from build123d import *

# Parameters (mm, degrees)
F0_W     = 100
F0_H     = 40
F1_DEPTH = 10
F2_R     = 5
F3_DEPTH = 10
F4_W     = 30
F4_H     = 40
F5_DEPTH = 10
F6_W     = 30
F6_H     = 20
F7_DEPTH = 10


with BuildPart() as f1:
    # F0 (on Top) → F1 (new body)
    with BuildSketch(Plane.XY):
        with Locations((40, 0)):
            Rectangle(F0_W, F0_H)
    extrude(amount=F1_DEPTH)

    # F2 (on face) → F3 (cut, through all)
    with BuildSketch(Plane.XY.offset(10)):
        Circle(F2_R)
    extrude(amount=-F3_DEPTH, mode=Mode.SUBTRACT)

    # F4 (on face) → F5 (join)
    with BuildSketch(Plane.XY.offset(10)):
        with Locations((75, 0)):
            Rectangle(F4_W, F4_H)
    extrude(amount=F5_DEPTH)

    # F6 (on face) → F7 (cut)
    with BuildSketch(Plane.XY.offset(20)):
        with Locations((75, 0)):
            Rectangle(F6_W, F6_H)
    extrude(amount=-F7_DEPTH, mode=Mode.SUBTRACT)


solid = f1.part
Can you work these out from the model? Positions are in its coordinate system, mm. A direction names the side the tool comes from. Give positions to 0.01 mm unless a question says otherwise; leave off trailing zeros. Loops run counter-clockwise (first coordinate to the right, second up) from the corner with the lowest first, then second, coordinate; pieces in that order, holes last. Notation, with made-up numbers: (6.25, 46) - (14.25, 46) arc R20 ccw to (14.25, 75) - close; hole circle Ø3 at (79, 20.5). An arc over 180 degrees is marked (long way). Return JSON: item names as keys, results as strings.
1. For faces 1 (the face through (-10, 0, 5)), 2 (the face through (75, -10, 15)), 3 (the face through (60, -15, 15)), which set-ups out of +Z, -Z, +X, -X, +Y, -Y let a thin tool reach every point of the face, with its end or its side?
Output values:
{"face 1": "+Z, -Z, -X, +Y, -Y", "face 2": "+Z, +X, -X", "face 3": "+Z, -X, +Y, -Y"}
2. I want a section at A-A on x = 4. Please give me the cut outline in (y, z), and give its area (3 significant figures).
Output values:
{"outline": "(-20, 0) - (-3, 0) - (-3, 10) - (-20, 10) - close; (3, 0) - (20, 0) - (20, 10) - (3, 10) - close", "area": "340 mm²"}
3. I want a section at B-B on y = 0. Please give me the cut outline in (x, z), and give its area (3 significant figures).
Output values:
{"outline": "(-10, 0) - (-5, 0) - (-5, 10) - (-10, 10) - close; (5, 0) - (90, 0) - (90, 10) - (5, 10) - close", "area": "900 mm²"}
4. I'm going to push flat-ended pins straight in: pin 1 Ø11.5 at (x, y) = (0, 0) entering from +Z; pin 2 Ø8 at (y, z) = (7.5, 14.5) entering from -X. Where does each tip first touch, or does it pass through?
Output values:
{"pin 1": "stops at z = 10", "pin 2": "stops at x = 60"}
5. If I drill on line 1 (Y direction, x = 0, z = 7.75); line 2 (Y direction, x = 63.5, z = 12.25); line 3 (Z direction, x = 76, y = -7.5), over which ranges is the centre line in solid material (lowest first)?
Output values:
{"line 1": "y = -20 to -5, 5 to 20", "line 2": "y = -20 to -10, 10 to 20", "line 3": "z = 0 to 10"}
6. We'd pull the mould along Y, two halves only. Please class faces 4 (the face through (-1.08, -4.88, 5.07)), 5 (the face through (75, -15, 20)), 6 (the face through (50, 20, 8)): +Y half, -Y half, draft (parallel to the pull), parting line (faces both ways), or undercut.
Output values:
{"face 4": "undercut", "face 5": "draft", "face 6": "+Y half"}
7. I want a section at D-D on x = 83. Please give me the cut outline in (y, z), and give its area (3 significant figures).
Output values:
{"outline": "(-20, 0) - (20, 0) - (20, 20) - (10, 20) - (10, 10) - (-10, 10) - (-10, 20) - (-20, 20) - close", "area": "600 mm²"}
8. I want a section at C-C on z = 4. Please give me the cut outline in (x, y), and give its area (3 significant figures).
Output values:
{"outline": "(-10, -20) - (90, -20) - (90, 20) - (-10, 20) - close; hole circle Ø10 at (0, 0)", "area": "3,920 mm²"}
